The listing builds one solid part. Answer for the finished solid, in the listing's coordinates (mm). A direction names the side the tool comes from. Give positions to 0.01 mm unless a question says otherwise; leave off trailing zeros. Order: outer loops, then holes, each group sorted by start corner. A loop starts at its lowest first (then second) coordinate and runs counter-clockwise, first axis right, second up. Notation, with made-up numbers: (86.25, 50) - (122.25, 50) arc R23 cw to (122.25, 79) - close; hole circle Ø2 at (75.25, 78). An arc over 180 degrees is marked (long way). Answer in a Markdown table with one row per item.
from build123d import *
from build123d.topology import SkipClean

# Parameters (mm, degrees)
EXTRUDE_1_DEPTH     = 1.5
CUT_EXTRUDE_1_DEPTH = 25.80423351
SKETCH_5_R          = 4
EXTRUDE_2_DEPTH     = 28.5
SKETCH_8_R          = 1.5
CUT_EXTRUDE_2_DEPTH = 10.5
CUT_EXTRUDE_3_DEPTH = 3
SKETCH_11_R         = 1.5
CUT_EXTRUDE_4_DEPTH = 5


with BuildPart() as part:
    # 草图1 → 凸台-拉伸1 (new, symmetric)
    with BuildSketch(Plane.XY):
        with BuildLine():
            Line((-4.5, 7.5), (4.5, 7.5))
            Line((4.5, 7.5), (4.5, 12))
            ThreePointArc((4.5, 12), (9.857189903, 10.7378078), (14.087412587, 7.216752724))
            ThreePointArc((14.087412587, 7.216752724), (16.191153731, 5.146301215), (18.807692308, 3.780203808))
            ThreePointArc((18.807692308, 3.780203808), (21.5, 0), (18.807692308, -3.780203808))
            ThreePointArc((18.807692308, -3.780203808), (16.191153731, -5.146301215), (14.087412587, -7.216752724))
            ThreePointArc((14.087412587, -7.216752724), (9.857189903, -10.7378078), (4.5, -12))
            Line((4.5, -12), (4.5, -7.5))
            Line((4.5, -7.5), (-4.5, -7.5))
            Line((-4.5, -7.5), (-4.5, -12))
            ThreePointArc((-4.5, -12), (-9.857189903, -10.7378078), (-14.087412587, -7.216752724))
            ThreePointArc((-14.087412587, -7.216752724), (-16.191153731, -5.146301215), (-18.807692308, -3.780203808))
            ThreePointArc((-18.807692308, -3.780203808), (-21.5, 0), (-18.807692308, 3.780203808))
            ThreePointArc((-18.807692308, 3.780203808), (-16.191153731, 5.146301215), (-14.087412587, 7.216752724))
            ThreePointArc((-14.087412587, 7.216752724), (-9.857189903, 10.7378078), (-4.5, 12))
            Line((-4.5, 12), (-4.5, 7.5))
        make_face()
    extrude(amount=EXTRUDE_1_DEPTH, both=True)

    # 草图4 → 切除-拉伸1 (cut, through all)
    with BuildSketch(Plane.XY.offset(1.5)):
        with BuildLine():
            Line((-4, 2.061552813), (-4, -2.061552813))
            ThreePointArc((-4, -2.061552813), (4.5, 0), (-4, 2.061552813))
        make_face()
    extrude(amount=-CUT_EXTRUDE_1_DEPTH, mode=Mode.SUBTRACT)

    # 草图5 → 凸台-拉伸2 (add)
    with BuildSketch(Plane(origin=(0, 0, -1.5), x_dir=(-1, 0, 0), z_dir=(0, 0, -1))):
        with Locations(Location((-17.5, 0, 0), (0, 0, 109.082124804))):
            Circle(SKETCH_5_R)
    extrude_2 = extrude(amount=EXTRUDE_2_DEPTH)

    # 草图8 → 切除-拉伸2 (cut)
    with BuildSketch(Plane(origin=(0, 0, -30), x_dir=(-1, 0, 0), z_dir=(0, 0, -1))):
        with Locations((-17.5, 0)):
            Circle(SKETCH_8_R)
    cut_extrude_2 = extrude(amount=-CUT_EXTRUDE_2_DEPTH, mode=Mode.SUBTRACT)

    # 镜向2: 凸台-拉伸2, 切除-拉伸2 across plane
    with SkipClean():  # the faces are left unmerged after this step: merging them gives an invalid solid
        add(extrude_2.mirror(Plane(origin=(0, 0, 0), x_dir=(0, 0, 1), z_dir=(1, 0, 0))))
        add(cut_extrude_2.mirror(Plane(origin=(0, 0, 0), x_dir=(0, 0, 1), z_dir=(1, 0, 0))), mode=Mode.SUBTRACT)

    # 草图10 → 切除-拉伸3 (cut, symmetric)
    with SkipClean():  # the faces are left unmerged after this step: merging them gives an invalid solid
        with BuildSketch(Plane(origin=(0, 0, -15.5), x_dir=(-1, 0, 0), z_dir=(0, 0, -1))):
            with BuildLine():
                Line((20.145751311, -3), (20.145751311, 3))
                ThreePointArc((20.145751311, 3), (21.5, 0), (20.145751311, -3))
            make_face()
        extrude(amount=CUT_EXTRUDE_3_DEPTH, both=True, mode=Mode.SUBTRACT)

    # 草图11 → 切除-拉伸4 (cut)
    with SkipClean():  # the faces are left unmerged after this step: merging them gives an invalid solid
        with BuildSketch(Plane.ZY.offset(20.145751311)):
            with Locations((-15.5, 0)):
                Circle(SKETCH_11_R)
        extrude(amount=-CUT_EXTRUDE_4_DEPTH, mode=Mode.SUBTRACT)


solid = part.part
Item 1: Find section A-A on x = 0. Write down the section's boundary in (y, z).
Answer block:
| item | result |
|---|---|
| outline | (-7.5, -1.5) - (-4.5, -1.5) - (-4.5, 1.5) - (-7.5, 1.5) - close; (4.5, -1.5) - (7.5, -1.5) - (7.5, 1.5) - (4.5, 1.5) - close |
Item 2: Each of these flat-tipped pins is pushed along its axis until it touches: P1, Ø2, axis at x = 15.5, z = -3, coming from the -Y side; P2, Ø1.5, axis at y = -10, z = 0, coming from the +X side; P3, Ø6, axis at x = 8.5, z = -26, coming from the +Y side; P4, Ø0.9, axis at y = -9.5, z = -0.5, coming from the -X side. Where does it stop, or does it pass through?
Answer block:
| item | result |
|---|---|
| P1 | y = -3.87 |
| P2 | x = 12.14 |
| P3 | through |
| P4 | x = -12.38 |
Item 3: Find section B-B on y = 0. Write down the section's boundary in (x, z).
Answer block:
| item | result |
|---|---|
| outline | (-21.5, -30) - (-19, -30) - (-19, -19.5) - (-16, -19.5) - (-16, -30) - (-13.5, -30) - (-13.5, -1.5) - (-4, -1.5) - (-4, 1.5) - (-21.5, 1.5) - (-21.5, -12.5) - (-20.15, -12.5) - (-20.15, -14) - (-15.15, -14) - (-15.15, -17) - (-20.15, -17) - (-20.15, -18.5) - (-21.5, -18.5) - close; (4.5, -1.5) - (13.5, -1.5) - (13.5, -30) - (16, -30) - (16, -19.5) - (19, -19.5) - (19, -30) - (21.5, -30) - (21.5, 1.5) - (4.5, 1.5) - close |
Item 4: Find section D-D on z = -3. Write down the section's boundary in (x, y).
Answer block:
| item | result |
|---|---|
| outline | circle Ø8 at (-17.5, 0); circle Ø8 at (17.5, 0) |
Item 5: Which of the six approach directions +Z, -Z, +X, -X, +Y, -Y give full straight-line access (tool end or side, diameter ignored) to faces 1 (the face through (-18, 0, -19.5)), 2 (the face through (-21, 0, -12.5)), 3 (the face through (-4, 0, 0))?
Answer block:
| item | result |
|---|---|
| face 1 | -Z |
| face 2 | -X, +Y, -Y |
| face 3 | +Z, -Z |
Item 6: Determine the mould class of faces 4 (the face through (-15.146, 0, -16)), 5 (the face through (4, 3, -1.5)), 6 (the face through (-9.79, -10.77, 0.02)), 7 (the face through (-19, 0, -25)) for opening direction Y: pulls with the +Y half, pulls with the -Y half, needs draft (parallel to the pull), parting line crosses it, or undercut.
Answer block:
| item | result |
|---|---|
| face 4 | undercut |
| face 5 | needs draft |
| face 6 | pulls with the -Y half |
| face 7 | undercut |
Item 7: Find section C-C on z = -24. Write down the section's boundary in (x, y), then the cut area to 3 significant figures.
Answer block:
| item | result |
|---|---|
| outline | circle Ø8 at (-17.5, 0); circle Ø8 at (17.5, 0); hole circle Ø3 at (-17.5, 0); hole circle Ø3 at (17.5, 0) |
| area | 86.4 mm² |
Item 8: Consider line 1 (Y direction, x = -17.5, z = -22.5); line 2 (Y direction, x = 0, z = 0); line 3 (Z direction, x = -6, y = 7). Determine where each line is inside the solid, lowest interval first.
Answer block:
| item | result |
|---|---|
| line 1 | -4 to -1.5, 1.5 to 4 |
| line 2 | -7.5 to -4.5, 4.5 to 7.5 |
| line 3 | -1.5 to 1.5 |
